from build123d import *

# Parameters (mm, degrees)
F1_DEPTH = 50
F3_DEPTH = 45


with BuildPart() as f1:
    # F0 (on Front) → F1 (new body)
    with BuildSketch(Plane.XZ):
        Polygon((35, 802.75), (35, 122.75), (965, 727.25), (965, 1407.25), align=None)
        Polygon((915, 756.371666), (85, 214.10179), (85, 775.615698), (915, 1315.115698), align=None, mode=Mode.SUBTRACT)
    extrude(amount=F1_DEPTH)

    # F2 (on face) → F3 (cut)
    with BuildSketch(Plane.XZ.offset(50)):
        Polygon((40, 800.03657), (40, 131.96343), (960, 729.96343), (960, 1398.03657), align=None)
    extrude(amount=-F3_DEPTH, mode=Mode.SUBTRACT)


solid = f1.part
Work out the finished part from the listing and answer in its coordinate system (mm). A direction names the side the tool comes from. Round coordinates to 2 decimals unless told otherwise and drop trailing zeros. Order: outer loops, then holes, each group sorted by start corner. A loop starts at its lowest first (then second) coordinate and runs counter-clockwise, first axis right, second up. Notation, with made-up numbers: M 84,67.25 L 130,67.25 A21 cw 130,76.25 Z; hole C 33.25,9 d1. An arc over 180 degrees is marked long. One line per item, written item: value.
Q1. Find section A-A on x = 244. Write down the section's boundary in (y, z).
Derived:
outline: M -50,258.6 L 0,258.6 L 0,317.98 L -5,317.98 L -5,264.56 L -50,264.56 Z; M -50,932.64 L -5,932.64 L -5,878.97 L 0,878.97 L 0,938.6 L -50,938.6 Z
Q2. Straight lines are drawn through the part: line 1 (X direction, y = -2.5, z = 767); line 2 (X direction, y = -21, z = 767); line 3 (Y direction, x = 100, z = 817). For each, find the intervals that lie inside material, in ascending order.
Derived:
line 1: 35 to 85, 915 to 965
line 2: 35 to 40, 960 to 965
line 3: -5 to 0
Q3. Find section C-C on z = 843. Write down the section's boundary in (x, y), then the cut area to 3 significant figures.
Derived:
outline: M 96.92,-50 L 106.1,-50 L 106.1,-5 L 188.67,-5 L 188.67,0 L 96.92,0 Z; M 915,-5 L 960,-5 L 960,-50 L 965,-50 L 965,0 L 915,0 Z
area: 1,350 mm²
Q4. Flat-ended cylindrical pins translate along their axes: pin 1 (1.5 mm diameter, centred on y = -3.5, z = 1092.5, fed in from -X); pin 2 (4 mm diameter, centred on x = 586, y = -22, fed in from +Z); pin 3 (4 mm diameter, centred on y = -3, z = 508.5, fed in from +X). Find the tip coordinate at first contact, or state that the pin passes through.
Derived:
pin 1: x = 479.62
pin 2: z = 1162.2
pin 3: x = 631.54
Q5. Determine the mould class of faces 1 (the face through (506.51, -24.65, 1109.23)), 2 (the face through (493.56, -27.815, 426.777)), 3 (the face through (965, -25, 1062)) for opening direction X: released by +X, released by -X, zero draft, split by the parting line, or undercut.
Derived:
face 1: released by -X
face 2: undercut
face 3: released by +X
Q6. Find section B-B on y = -36. Write down the section's boundary in (x, z), then the cut area to 3 significant figures.
Derived:
outline: M 35,122.75 L 965,727.25 L 965,1407.25 L 35,802.75 Z; hole M 40,131.96 L 960,729.96 L 960,1398.04 L 40,800.04 Z
area: 17,800 mm²
Q7. For faces 4 (the face through (506.44, -27.815, 1103.223)), 5 (the face through (505.81, -2.465, 489.033)), 6 (the face through (35, -25, 468)), determine the directions among +Z, -Z, +X, -X, +Y, -Y from which every point of the face is accessible in a straight line to the end or side of a thin tool.
Derived:
face 4: -Y
face 5: +Y, -Y
face 6: +Z, -Z, -X, +Y, -Y
